from build123d import *

# Parameters (mm, degrees)
F0_W     = 50.8
F0_H     = 50.8
F1_DEPTH = 50.8
F2_R     = 7.4453677319
F3_DEPTH = 50.8
F5_DEPTH = 4.7625
F6_R     = 1.5875
F7_DEPTH = 25.4


with BuildPart() as f1:
    # F0 (on Front) → F1 (new body)
    with BuildSketch(Plane.XZ):
        with Locations((-0.097932294, -5.0924364477)):
            Rectangle(F0_W, F0_H)
    extrude(amount=F1_DEPTH)

    # F2 (on face) → F3 (cut)
    with BuildSketch(Plane.XZ.offset(50.8)):
        with Locations((0, -10.2828023955)):
            Circle(F2_R)
    extrude(amount=-F3_DEPTH, mode=Mode.SUBTRACT)


with BuildPart() as f5:
    # F4 (on Top) → F5 (new body)
    with BuildSketch(Plane.XY):
        Polygon((-51.9754371398, 50.3634488253), (-47.8477183507, 52.7390211454), (-47.8411649339, 57.5015166365), (-51.9623303063, 59.8884398075), (-56.0900490953, 57.5128674873), (-56.0966025121, 52.7503719962), align=None)
    extrude(amount=F5_DEPTH)

    # F5_face (on face) + F6 (on face) → F7 (cut)
    with BuildSketch(Plane(origin=(-51.968883723, 55.1259443164, 4.7625), x_dir=(1, 0, 0), z_dir=(0, 0, 1))):
        Polygon((-0.0065534168, -4.7624954911), (4.1211653723, -2.3869231709), (4.1277187891, 2.3755723202), (0.0065534168, 4.7624954911), (-4.1211653723, 2.3869231709), (-4.1277187891, -2.3755723202), align=None)
    with BuildSketch(Plane.XY):
        with Locations((-51.968883723, 55.1259443164)):
            Circle(F6_R)
    extrude(amount=-F7_DEPTH, mode=Mode.SUBTRACT)


solid = f1.part
Work out the finished part from the listing and answer in its coordinate system (mm). Give positions to 0.01 mm unless a question says otherwise; leave off trailing zeros. Write each loop counter-clockwise with the first axis right and the second up, starting at its lowest first coordinate (ties: lowest second). Pieces come first, ordered by that corner, then holes.
Q1. Straight lines are drawn through the part: L1, parallel to X at y = -29.5, z = -10; L2, parallel to Z at x = 0, y = -29; L3, parallel to Z at x = 3.5, y = -1.5. For each, find the intervals that lie inside material, in ascending order.
Answer:
L1: x = -25.5 to -7.44, 7.44 to 25.3
L2: z = -30.49 to -17.73, -2.84 to 20.31
L3: z = -30.49 to -16.85, -3.71 to 20.31
Q2. The part is cut by section A-A on x = 0. Give the vertices of the cut face in (y, z), and give its area (3 significant figures).
Answer:
outline: (-50.8, -30.49) - (0, -30.49) - (0, -17.73) - (-50.8, -17.73) - close; (-50.8, -2.84) - (0, -2.84) - (0, 20.31) - (-50.8, 20.31) - close
area: 1,820 mm2
Q3. For a pull along Z with two mould halves and no side action, classify faces 1 (the face through (-25.498, -25, -5)), 2 (the face through (0, -25, 20.308)), 3 (the face through (3.436, -25.756, -16.888)) as released by +Z, released by -Z, zero draft, split by the parting line, or undercut.
Answer:
face 1: zero draft
face 2: released by +Z
face 3: undercut
Q4. The part is cut by section C-C on y = -38. Give the vertices of the cut face in (x, z), and give its area (3 significant figures).
Answer:
outline: (-25.5, -30.49) - (25.3, -30.49) - (25.3, 20.31) - (-25.5, 20.31) - close; hole circle Ø14.89 at (0, -10.28)
area: 2,410 mm2
Q5. The part is cut by section B-B on z = -15. Give the vertices of the cut face in (x, y).
Answer:
outline: (-25.5, -50.8) - (-5.76, -50.8) - (-5.76, 0) - (-25.5, 0) - close; (5.76, -50.8) - (25.3, -50.8) - (25.3, 0) - (5.76, 0) - close
